```python
from build123d import *

# Parameters (mm, degrees)
EXTRUDE_1_DEPTH     = 5
SKETCH_2_R          = 2.5
CUT_EXTRUDE_1_DEPTH = 10
SKETCH_3_R          = 20
CUT_EXTRUDE_2_DEPTH = 256.697575272
CUT_EXTRUDE_3_DEPTH = 256.697575272
SKETCH_5_R          = 1.6
CUT_EXTRUDE_4_DEPTH = 256.697575272
SKETCH_6_R          = 2.1
CUT_EXTRUDE_5_DEPTH = 256.697575272


with BuildPart() as part:
    # 草图1 → 凸台-拉伸1 (new body)
    with BuildSketch(Plane.XY):
        with BuildLine():
            Line((-212.5, 40), (212.5, 40))
            ThreePointArc((212.5, 40), (252.5, 0), (212.5, -40))
            Line((212.5, -40), (-212.5, -40))
            ThreePointArc((-212.5, -40), (-252.5, 0), (-212.5, 40))
        make_face()
    extrude(amount=EXTRUDE_1_DEPTH)

    # 草图2 → 切除-拉伸1 (cut)
    with BuildSketch(Plane.XY.offset(5)):
        with Locations((-7.5, 30)):
            Circle(SKETCH_2_R)
        with Locations((7.5, 30)):
            Circle(SKETCH_2_R)
        with Locations((7.5, -30)):
            Circle(SKETCH_2_R)
        with Locations((-7.5, -30)):
            Circle(SKETCH_2_R)
    extrude(amount=-CUT_EXTRUDE_1_DEPTH, mode=Mode.SUBTRACT)

    # 草图3 → 切除-拉伸2 (cut, through all)
    with BuildSketch(Plane.XY.offset(5)):
        with Locations((-212.5, 0)):
            Circle(SKETCH_3_R)
        with Locations((212.5, 0)):
            Circle(SKETCH_3_R)
    extrude(amount=-CUT_EXTRUDE_2_DEPTH, mode=Mode.SUBTRACT)

    # 草图4 → 切除-拉伸3 (cut, through all)
    with BuildSketch(Plane(origin=(0, 0, 0), x_dir=(-1, 0, 0), z_dir=(0, 0, -1))):
        with BuildLine():
            Line((-16.665194888, -12.934457925), (-16.665194888, -19.318378476))
            ThreePointArc((-16.665194888, -19.318378476), (-21.665194888, -24.318378476), (-26.665194888, -19.318378476))
            Line((-26.665194888, -19.318378476), (-26.665194888, -12.934457925))
            ThreePointArc((-26.665194888, -12.934457925), (-21.665194888, -7.934457925), (-16.665194888, -12.934457925))
        make_face()
        with BuildLine():
            Line((26.665194888, 19.318378476), (26.665194888, 12.934457925))
            ThreePointArc((26.665194888, 12.934457925), (21.665194888, 7.934457925), (16.665194888, 12.934457925))
            Line((16.665194888, 12.934457925), (16.665194888, 19.318378476))
            ThreePointArc((16.665194888, 19.318378476), (21.665194888, 24.318378476), (26.665194888, 19.318378476))
        make_face()
    extrude(amount=-CUT_EXTRUDE_3_DEPTH, mode=Mode.SUBTRACT)

    # 草图5 → 切除-拉伸4 (cut, through all)
    with BuildSketch(Plane.XY.offset(5)):
        with Locations((57.5, -25)):
            Circle(SKETCH_5_R)
        with Locations((77.5, -25)):
            Circle(SKETCH_5_R)
        with Locations((97.5, -25)):
            Circle(SKETCH_5_R)
        with Locations((117.5, -25)):
            Circle(SKETCH_5_R)
        with Locations((137.5, -25)):
            Circle(SKETCH_5_R)
        with Locations((157.5, -25)):
            Circle(SKETCH_5_R)
        with Locations((-57.5, 25)):
            Circle(SKETCH_5_R)
        with Locations((-77.5, 25)):
            Circle(SKETCH_5_R)
        with Locations((-97.5, 25)):
            Circle(SKETCH_5_R)
        with Locations((-117.5, 25)):
            Circle(SKETCH_5_R)
        with Locations((-137.5, 25)):
            Circle(SKETCH_5_R)
        with Locations((-157.5, 25)):
            Circle(SKETCH_5_R)
    extrude(amount=-CUT_EXTRUDE_4_DEPTH, mode=Mode.SUBTRACT)

    # 草图6 → 切除-拉伸5 (cut, through all)
    with BuildSketch(Plane(origin=(0, 0, 0), x_dir=(-1, 0, 0), z_dir=(0, 0, -1))):
        with Locations((-247.5, 0)):
            Circle(SKETCH_6_R)
        with Locations((-237.248737342, 24.748737342)):
            Circle(SKETCH_6_R)
        with Locations((-212.5, 35)):
            Circle(SKETCH_6_R)
        with Locations((-187.751262658, 24.748737342)):
            Circle(SKETCH_6_R)
        with Locations((-177.5, 0)):
            Circle(SKETCH_6_R)
        with Locations((-187.751262658, -24.748737342)):
            Circle(SKETCH_6_R)
        with Locations((-212.5, -35)):
            Circle(SKETCH_6_R)
        with Locations((-237.248737342, -24.748737342)):
            Circle(SKETCH_6_R)
    cut_extrude_5 = extrude(amount=-CUT_EXTRUDE_5_DEPTH, mode=Mode.SUBTRACT)

    # 镜向1: 切除-拉伸5 across plane
    add(cut_extrude_5.mirror(Plane(origin=(0, 0, 0), x_dir=(0, 0, 1), z_dir=(1, 0, 0))), mode=Mode.SUBTRACT)


solid = part.part
```
Check sheet for the modelled part. Datum: model origin and axes. Units: mm. Coordinates: 2 decimals unless noted, no trailing zeros. Write item = value, one per line. Start each with the question number.
1. Sectioned sample at A-A (z = 2.55). State how many separate pieces and enclosed holes the cut face has, then the cut area to 3 significant figures.
2. Thickness scan on probe 1 along Y at (x, z) = (-212.5, 3.8); probe 2 along Y at (x, z) = (-247.5, 3.25); probe 3 along Y at (x, z) = (-117.5, 2.5). Record the ranges inside material, lowest first.
3. Go/stop test with a flat-tipped pin: pin 1 (1.5 mm diameter, centred on y = 27, z = 4.5, fed in from +X). Record where the tip stops, or that it passes through.
The answers:
q1.separate_pieces = 1
q1.enclosed_holes = 36
q1.area = 35,800 mm²
q2.probe_1 = -40 to -37.1, -32.9 to -20, 20 to 32.9, 37.1 to 40
q2.probe_2 = -19.36 to -2.1, 2.1 to 19.36
q2.probe_3 = -40 to 23.4, 26.6 to 40
q3.pin_1 = 242.68
